Verification items for this drawing (mm, ordinates from the low corner). A direction names the side the tool comes from. Round coordinates to 2 decimals unless told otherwise and drop trailing zeros. Order: outer loops, then holes, each group sorted by start corner. A loop starts at its lowest first (then second) coordinate and runs counter-clockwise, first axis right, second up. Notation, with made-up numbers: (63, 58) - (115, 58) arc R9 cw to (115, 69) - close; hole circle Ø10 at (77, 25). An arc over 180 degrees is marked (long way). Use a Markdown table: item, result. Add a question column.
(1) Section check A-A on x = 2.5. Record the boundary of the cut face in (y, z).
(2) Section check D-D on x = 1.7. Record the boundary of the cut face in (y, z).
(3) Section check C-C on y = 2.25. Record the boundary of the cut face in (x, z).
(4) Thickness scan on line 1 along Z through (x, y) = (4.55, 3.5); line 2 along Y through (x, z) = (3, 2.25); line 3 along Y through (x, z) = (2.5, 9.05). Record the ranges inside material, lowest first. Write a range as [from, to].
(5) Mould release check, pull along X, two halves, no side actions. Record for the marked faces 1, 2, 3 and 4: released by +X, released by -X, zero draft, split by the parting line, or undercut.
(6) Gauge pin test, flat ends, axial feed: P1, Ø2.5, axis at x = 2, y = 1.5, coming from the -Z side; P2, Ø0.6, axis at x = 4.5, y = 6.5, coming from the -Z side; P3, Ø3, axis at x = 2.5, z = 1, coming from the -Y side. Record the tip position at first contact, or that the pin passes through.
(7) Access from +Z, -Z, +X, -X, +Y, -Y to the whole of each face (thin tool, end or side, straight path). Record for the marked faces 5 and 6.
(8) Section check B-B on z = 2. Record the boundary of the cut face in (x, y) (1 decimal).
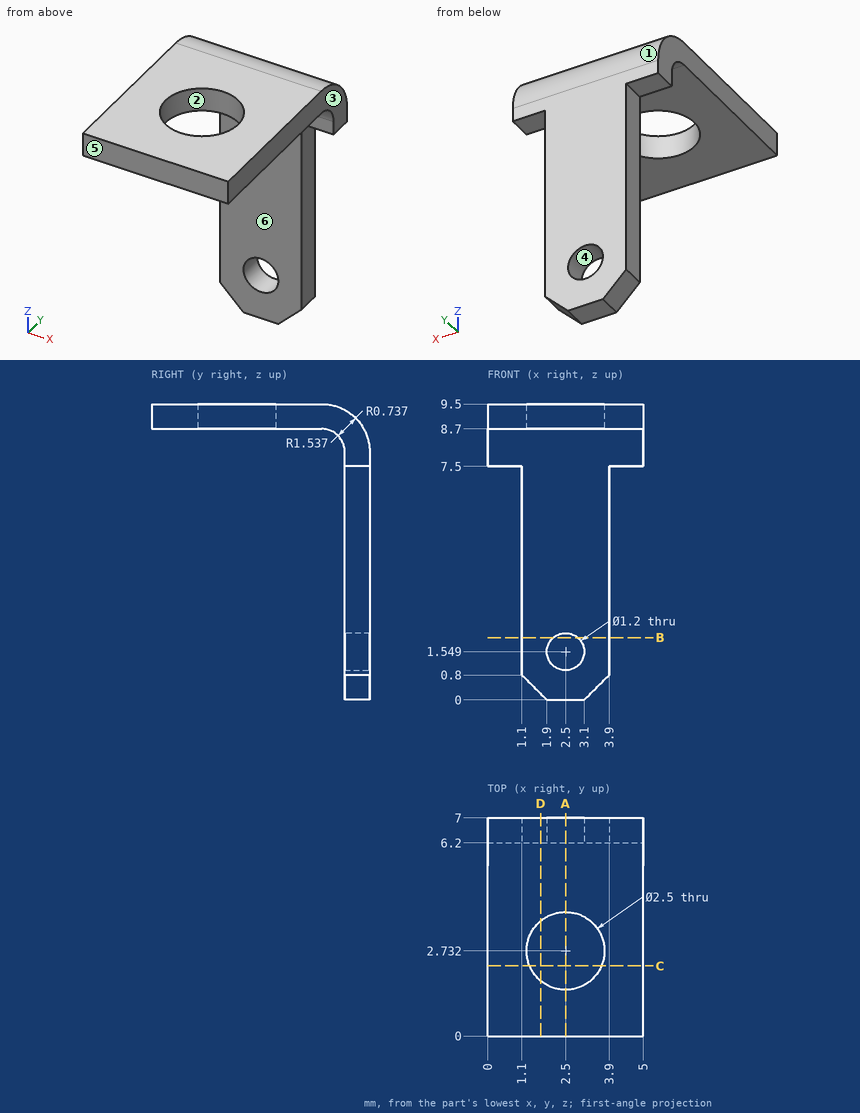
Check sheet entries:
| question | item | result |
|---|---|---|
| 1 | outline | (0, 8.7) - (1.48, 8.7) - (1.48, 9.5) - (0, 9.5) - close; (3.98, 8.7) - (5.46, 8.7) arc R0.74 cw to (6.2, 7.96) - (6.2, 2.15) - (7, 2.15) - (7, 7.96) arc R1.54 ccw to (5.46, 9.5) - (3.98, 9.5) - close; (6.2, 0) - (7, 0) - (7, 0.95) - (6.2, 0.95) - close |
| 2 | outline | (0, 8.7) - (1.77, 8.7) - (1.77, 9.5) - (0, 9.5) - close; (3.69, 8.7) - (5.46, 8.7) arc R0.74 cw to (6.2, 7.96) - (6.2, 0.2) - (7, 0.2) - (7, 7.96) arc R1.54 ccw to (5.46, 9.5) - (3.69, 9.5) - close |
| 3 | outline | (0, 8.7) - (1.35, 8.7) - (1.35, 9.5) - (0, 9.5) - close; (3.65, 8.7) - (5, 8.7) - (5, 9.5) - (3.65, 9.5) - close |
| 4 | line 1 | z = [8.7, 9.5] |
| 4 | line 2 | y = [6.2, 7] |
| 4 | line 3 | y = [0, 1.48], [3.98, 6.55] |
| 5 | face 1 | zero draft |
| 5 | face 2 | undercut |
| 5 | face 3 | released by +X |
| 5 | face 4 | undercut |
| 6 | P1 | stops at z = 8.7 |
| 6 | P2 | stops at z = 7.5 |
| 6 | P3 | stops at y = 6.2 |
| 7 | face 5 | +Z, -Z, +X, -X, -Y |
| 7 | face 6 | -Z, +X, -X, -Y |
| 8 | outline | (1.1, 6.2) - (2.1, 6.2) - (2.1, 7) - (1.1, 7) - close; (2.9, 6.2) - (3.9, 6.2) - (3.9, 7) - (2.9, 7) - close |
